Check sheet for the modelled part. Datum: model origin and axes. Units: mm. Give positions to 0.01 mm unless a question says otherwise; leave off trailing zeros. Order: outer loops, then holes, each group sorted by start corner. A loop starts at its lowest first (then second) coordinate and runs counter-clockwise, first axis right, second up. Notation, with made-up numbers: (-3.5, 54) -> (42.5, 54) arc R15 ccw to (42.5, 72) -> close; hole circle Ø3 at (7.25, 43). An arc over 180 degrees is marked (long way). Write each question's results on one line, items separated by ' | '.
from build123d import *

# Parameters (mm, degrees)
SKETCH8_W           = 113.299968811
SKETCH8_H           = 61.218531535
BOSS_EXTRUDE6_DEPTH = 10
FILLET7_R           = 10


with BuildPart() as part:
    # Sketch8 → Boss-Extrude6 (new body)
    with BuildSketch(Plane.XY):
        with Locations((-35.943575618, 24.354623855)):
            Rectangle(SKETCH8_W, SKETCH8_H)
    extrude(amount=BOSS_EXTRUDE6_DEPTH)

    # Fillet7
    fillet7_edges = [part.edges().sort_by_distance(p)[0] for p in [
        (-35.943575617, 54.963889622, 0),
    ]]
    fillet(fillet7_edges, radius=FILLET7_R - 0.0001)  # a hair under: the kernel refuses the full size


solid = part.part
1. Gauge pin test, flat end, axial feed: pin 1 Ø1.5 at (x, z) = (-38, 2.5) entering from +Y. Record the tip position at first contact, or that the pin passes through.
Verdict:
pin 1: stops at y = 52.34
2. Material ranges on probe 1 along Y at (x, z) = (-64.5, 4.25); probe 2 along Y at (x, z) = (-30.5, 7.75); probe 3 along Z at (x, y) = (5, 51), recorded low to high. Write a range as from..to.
Verdict:
probe 1: y = -6.25..53.15 | probe 2: y = -6.25..54.71 | probe 3: z = 2.03..10
3. Section check B-B on y = 47.5. Record the cut outline in (x, z).
Verdict:
outline: (-92.59, 0.33) -> (20.71, 0.33) -> (20.71, 10) -> (-92.59, 10) -> close
4. Section check C-C on z = 4.5. Record the cut outline in (x, y), then the cut area to 3 significant figures.
Verdict:
outline: (-92.59, -6.25) -> (20.71, -6.25) -> (20.71, 53.32) -> (-92.59, 53.32) -> close | area: 6,750 mm^2
